```python
from build123d import *

# Parameters (mm, degrees)
SKETCH_1_R      = 1.7
SKETCH_1_R_2    = 2.5
SKETCH_1_R_3    = 2
EXTRUDE_2_DEPTH = 5


with BuildPart() as part:
    # 草图1 → 凸台-拉伸2 (new body)
    with BuildSketch(Plane(origin=(0, 0, 0), x_dir=(1, 0, 0), z_dir=(0, 1, 0))):
        with BuildLine():
            ThreePointArc((-65, 170), (-68.535533906, 168.535533906), (-70, 165))
            Line((-70, 165), (-70, 130))
            Line((-70, 130), (-70, -165))
            ThreePointArc((-70, -165), (-68.535533906, -168.535533906), (-65, -170))
            Line((-65, -170), (65, -170))
            ThreePointArc((65, -170), (68.535533906, -168.535533906), (70, -165))
            Line((70, -165), (70, 165))
            ThreePointArc((70, 165), (68.535533906, 168.535533906), (65, 170))
            Line((65, 170), (0, 170))
            Line((0, 170), (-65, 170))
        make_face()
        with Locations(Location((-62, -158, 0), (0, 0, 270))):
            Circle(SKETCH_1_R, mode=Mode.SUBTRACT)
        with Locations(Location((-48, -158, 0), (0, 0, 270))):
            Circle(SKETCH_1_R, mode=Mode.SUBTRACT)
        with Locations(Location((-62, -142, 0), (0, 0, 270))):
            Circle(SKETCH_1_R, mode=Mode.SUBTRACT)
        with Locations(Location((-48, -142, 0), (0, 0, 270))):
            Circle(SKETCH_1_R, mode=Mode.SUBTRACT)
        with Locations(Location((-35, -160, 0), (0, 0, 270))):
            Circle(SKETCH_1_R_2, mode=Mode.SUBTRACT)
        with Locations(Location((-60, -120, 0), (0, 0, 270))):
            Circle(SKETCH_1_R_3, mode=Mode.SUBTRACT)
        with Locations(Location((-60, -100, 0), (0, 0, 270))):
            Circle(SKETCH_1_R_3, mode=Mode.SUBTRACT)
        with Locations(Location((-40, -100, 0), (0, 0, 270))):
            Circle(SKETCH_1_R_3, mode=Mode.SUBTRACT)
        with Locations(Location((-20, -100, 0), (0, 0, 270))):
            Circle(SKETCH_1_R_3, mode=Mode.SUBTRACT)
        with Locations(Location((-60, -80, 0), (0, 0, 270))):
            Circle(SKETCH_1_R_3, mode=Mode.SUBTRACT)
        with Locations(Location((-60, -60, 0), (0, 0, 270))):
            Circle(SKETCH_1_R_3, mode=Mode.SUBTRACT)
        with Locations(Location((-40, -80, 0), (0, 0, 270))):
            Circle(SKETCH_1_R_3, mode=Mode.SUBTRACT)
        with Locations(Location((-40, -60, 0), (0, 0, 270))):
            Circle(SKETCH_1_R_3, mode=Mode.SUBTRACT)
        with Locations(Location((-60, -40, 0), (0, 0, 270))):
            Circle(SKETCH_1_R_3, mode=Mode.SUBTRACT)
        with Locations(Location((-60, -20, 0), (0, 0, 270))):
            Circle(SKETCH_1_R_3, mode=Mode.SUBTRACT)
        with Locations(Location((-60, 0, 0), (0, 0, 270))):
            Circle(SKETCH_1_R_3, mode=Mode.SUBTRACT)
        with Locations(Location((-40, -40, 0), (0, 0, 270))):
            Circle(SKETCH_1_R_3, mode=Mode.SUBTRACT)
        with Locations(Location((-20, -80, 0), (0, 0, 270))):
            Circle(SKETCH_1_R_3, mode=Mode.SUBTRACT)
        with Locations(Location((-20, -60, 0), (0, 0, 270))):
            Circle(SKETCH_1_R_3, mode=Mode.SUBTRACT)
        with Locations(Location((-20, -40, 0), (0, 0, 270))):
            Circle(SKETCH_1_R_3, mode=Mode.SUBTRACT)
        with BuildLine():
            Line((25, -140), (25, -160))
            ThreePointArc((25, -160), (23.535533906, -163.535533906), (20, -165))
            Line((20, -165), (-20, -165))
            ThreePointArc((-20, -165), (-23.535533906, -163.535533906), (-25, -160))
            Line((-25, -160), (-25, -140))
            ThreePointArc((-25, -140), (-23.535533906, -136.464466094), (-20, -135))
            Line((-20, -135), (20, -135))
            ThreePointArc((20, -135), (23.535533906, -136.464466094), (25, -140))
        make_face(mode=Mode.SUBTRACT)
        with Locations(Location((0, -100, 0), (0, 0, 270))):
            Circle(SKETCH_1_R_3, mode=Mode.SUBTRACT)
        with Locations(Location((20, -100, 0), (0, 0, 270))):
            Circle(SKETCH_1_R_3, mode=Mode.SUBTRACT)
        with Locations(Location((35, -160, 0), (0, 0, 270))):
            Circle(SKETCH_1_R_2, mode=Mode.SUBTRACT)
        with Locations(Location((48, -158, 0), (0, 0, 270))):
            Circle(SKETCH_1_R, mode=Mode.SUBTRACT)
        with Locations(Location((62, -158, 0), (0, 0, 270))):
            Circle(SKETCH_1_R, mode=Mode.SUBTRACT)
        with Locations(Location((48, -142, 0), (0, 0, 270))):
            Circle(SKETCH_1_R, mode=Mode.SUBTRACT)
        with Locations(Location((62, -142, 0), (0, 0, 270))):
            Circle(SKETCH_1_R, mode=Mode.SUBTRACT)
        with Locations(Location((40, -100, 0), (0, 0, 270))):
            Circle(SKETCH_1_R_3, mode=Mode.SUBTRACT)
        with Locations(Location((60, -120, 0), (0, 0, 270))):
            Circle(SKETCH_1_R_3, mode=Mode.SUBTRACT)
        with Locations(Location((60, -100, 0), (0, 0, 270))):
            Circle(SKETCH_1_R_3, mode=Mode.SUBTRACT)
        with Locations(Location((0, -80, 0), (0, 0, 270))):
            Circle(SKETCH_1_R_3, mode=Mode.SUBTRACT)
        with Locations(Location((0, -60, 0), (0, 0, 270))):
            Circle(SKETCH_1_R_3, mode=Mode.SUBTRACT)
        with Locations(Location((20, -80, 0), (0, 0, 270))):
            Circle(SKETCH_1_R_3, mode=Mode.SUBTRACT)
        with Locations(Location((20, -60, 0), (0, 0, 270))):
            Circle(SKETCH_1_R_3, mode=Mode.SUBTRACT)
        with Locations(Location((0, -40, 0), (0, 0, 270))):
            Circle(SKETCH_1_R_3, mode=Mode.SUBTRACT)
        with Locations(Location((20, -40, 0), (0, 0, 270))):
            Circle(SKETCH_1_R_3, mode=Mode.SUBTRACT)
        with Locations(Location((40, -80, 0), (0, 0, 270))):
            Circle(SKETCH_1_R_3, mode=Mode.SUBTRACT)
        with Locations(Location((40, -60, 0), (0, 0, 270))):
            Circle(SKETCH_1_R_3, mode=Mode.SUBTRACT)
        with Locations(Location((60, -80, 0), (0, 0, 270))):
            Circle(SKETCH_1_R_3, mode=Mode.SUBTRACT)
        with Locations(Location((60, -60, 0), (0, 0, 270))):
            Circle(SKETCH_1_R_3, mode=Mode.SUBTRACT)
        with Locations(Location((40, -40, 0), (0, 0, 270))):
            Circle(SKETCH_1_R_3, mode=Mode.SUBTRACT)
        with Locations(Location((60, -40, 0), (0, 0, 270))):
            Circle(SKETCH_1_R_3, mode=Mode.SUBTRACT)
        with Locations(Location((60, -20, 0), (0, 0, 270))):
            Circle(SKETCH_1_R_3, mode=Mode.SUBTRACT)
        with Locations(Location((-60, 20, 0), (0, 0, 270))):
            Circle(SKETCH_1_R_3, mode=Mode.SUBTRACT)
        with Locations(Location((-60, 40, 0), (0, 0, 270))):
            Circle(SKETCH_1_R_3, mode=Mode.SUBTRACT)
        with Locations(Location((-40, 40, 0), (0, 0, 270))):
            Circle(SKETCH_1_R_3, mode=Mode.SUBTRACT)
        with Locations(Location((-60, 60, 0), (0, 0, 270))):
            Circle(SKETCH_1_R_3, mode=Mode.SUBTRACT)
        with Locations(Location((-60, 80, 0), (0, 0, 270))):
            Circle(SKETCH_1_R_3, mode=Mode.SUBTRACT)
        with Locations(Location((-40, 60, 0), (0, 0, 270))):
            Circle(SKETCH_1_R_3, mode=Mode.SUBTRACT)
        with Locations(Location((-40, 80, 0), (0, 0, 270))):
            Circle(SKETCH_1_R_3, mode=Mode.SUBTRACT)
        with Locations(Location((-20, 40, 0), (0, 0, 270))):
            Circle(SKETCH_1_R_3, mode=Mode.SUBTRACT)
        with Locations(Location((-20, 60, 0), (0, 0, 270))):
            Circle(SKETCH_1_R_3, mode=Mode.SUBTRACT)
        with Locations(Location((-20, 80, 0), (0, 0, 270))):
            Circle(SKETCH_1_R_3, mode=Mode.SUBTRACT)
        with Locations(Location((-60, 100, 0), (0, 0, 270))):
            Circle(SKETCH_1_R_3, mode=Mode.SUBTRACT)
        with Locations(Location((-60, 120, 0), (0, 0, 270))):
            Circle(SKETCH_1_R_3, mode=Mode.SUBTRACT)
        with Locations(Location((-40, 100, 0), (0, 0, 270))):
            Circle(SKETCH_1_R_3, mode=Mode.SUBTRACT)
        with Locations(Location((-62, 142, 0), (0, 0, 270))):
            Circle(SKETCH_1_R, mode=Mode.SUBTRACT)
        with Locations(Location((-48, 142, 0), (0, 0, 270))):
            Circle(SKETCH_1_R, mode=Mode.SUBTRACT)
        with Locations(Location((-62, 158, 0), (0, 0, 270))):
            Circle(SKETCH_1_R, mode=Mode.SUBTRACT)
        with Locations(Location((-48, 158, 0), (0, 0, 270))):
            Circle(SKETCH_1_R, mode=Mode.SUBTRACT)
        with Locations(Location((-35, 160, 0), (0, 0, 270))):
            Circle(SKETCH_1_R_2, mode=Mode.SUBTRACT)
        with Locations(Location((-20, 100, 0), (0, 0, 270))):
            Circle(SKETCH_1_R_3, mode=Mode.SUBTRACT)
        with Locations(Location((0, 40, 0), (0, 0, 270))):
            Circle(SKETCH_1_R_3, mode=Mode.SUBTRACT)
        with Locations(Location((20, 40, 0), (0, 0, 270))):
            Circle(SKETCH_1_R_3, mode=Mode.SUBTRACT)
        with Locations(Location((0, 60, 0), (0, 0, 270))):
            Circle(SKETCH_1_R_3, mode=Mode.SUBTRACT)
        with Locations(Location((0, 80, 0), (0, 0, 270))):
            Circle(SKETCH_1_R_3, mode=Mode.SUBTRACT)
        with Locations(Location((20, 60, 0), (0, 0, 270))):
            Circle(SKETCH_1_R_3, mode=Mode.SUBTRACT)
        with Locations(Location((20, 80, 0), (0, 0, 270))):
            Circle(SKETCH_1_R_3, mode=Mode.SUBTRACT)
        with Locations(Location((40, 40, 0), (0, 0, 270))):
            Circle(SKETCH_1_R_3, mode=Mode.SUBTRACT)
        with Locations(Location((60, 0, 0), (0, 0, 270))):
            Circle(SKETCH_1_R_3, mode=Mode.SUBTRACT)
        with Locations(Location((60, 20, 0), (0, 0, 270))):
            Circle(SKETCH_1_R_3, mode=Mode.SUBTRACT)
        with Locations(Location((60, 40, 0), (0, 0, 270))):
            Circle(SKETCH_1_R_3, mode=Mode.SUBTRACT)
        with Locations(Location((40, 60, 0), (0, 0, 270))):
            Circle(SKETCH_1_R_3, mode=Mode.SUBTRACT)
        with Locations(Location((40, 80, 0), (0, 0, 270))):
            Circle(SKETCH_1_R_3, mode=Mode.SUBTRACT)
        with Locations(Location((60, 60, 0), (0, 0, 270))):
            Circle(SKETCH_1_R_3, mode=Mode.SUBTRACT)
        with Locations(Location((60, 80, 0), (0, 0, 270))):
            Circle(SKETCH_1_R_3, mode=Mode.SUBTRACT)
        with Locations(Location((0, 100, 0), (0, 0, 270))):
            Circle(SKETCH_1_R_3, mode=Mode.SUBTRACT)
        with Locations(Location((20, 100, 0), (0, 0, 270))):
            Circle(SKETCH_1_R_3, mode=Mode.SUBTRACT)
        with BuildLine():
            Line((-20, 165), (0, 165))
            Line((0, 165), (20, 165))
            ThreePointArc((20, 165), (23.535533906, 163.535533906), (25, 160))
            Line((25, 160), (25, 140))
            ThreePointArc((25, 140), (23.535533906, 136.464466094), (20, 135))
            Line((20, 135), (-20, 135))
            ThreePointArc((-20, 135), (-23.535533906, 136.464466094), (-25, 140))
            Line((-25, 140), (-25, 160))
            ThreePointArc((-25, 160), (-23.535533906, 163.535533906), (-20, 165))
        make_face(mode=Mode.SUBTRACT)
        with Locations(Location((40, 100, 0), (0, 0, 270))):
            Circle(SKETCH_1_R_3, mode=Mode.SUBTRACT)
        with Locations(Location((60, 100, 0), (0, 0, 270))):
            Circle(SKETCH_1_R_3, mode=Mode.SUBTRACT)
        with Locations(Location((60, 120, 0), (0, 0, 270))):
            Circle(SKETCH_1_R_3, mode=Mode.SUBTRACT)
        with Locations(Location((35, 160, 0), (0, 0, 270))):
            Circle(SKETCH_1_R_2, mode=Mode.SUBTRACT)
        with Locations(Location((48, 142, 0), (0, 0, 270))):
            Circle(SKETCH_1_R, mode=Mode.SUBTRACT)
        with Locations(Location((62, 142, 0), (0, 0, 270))):
            Circle(SKETCH_1_R, mode=Mode.SUBTRACT)
        with Locations(Location((48, 158, 0), (0, 0, 270))):
            Circle(SKETCH_1_R, mode=Mode.SUBTRACT)
        with Locations(Location((62, 158, 0), (0, 0, 270))):
            Circle(SKETCH_1_R, mode=Mode.SUBTRACT)
    extrude(amount=EXTRUDE_2_DEPTH)


solid = part.part
```
Verification items for the finished model (mm, model axes). Coordinates: 2 decimals unless noted, no trailing zeros. Put each result on its own line as item: value.
Item 1: Section check A-A (y = 1.8). Give the number of separate pieces and of enclosed holes in the cut face, then the cut area to 3 significant figures.
Conclusion:
separate pieces: 1
enclosed holes: 88
area: 43,600 mm2
Item 2: Scan lines: line 1 along X through (y, z) = (2.9, 160); line 2 along Z through (x, y) = (14, 2.3); line 3 along X through (y, z) = (2.1, 120). Record each from-to range of solid material in increasing order.
Conclusion:
line 1: x = -70 to -37.5, -32.5 to -25, 25 to 32.5, 37.5 to 70
line 2: z = -170 to -165, -135 to 135, 165 to 170
line 3: x = -70 to -62, -58 to 58, 62 to 70
Item 3: Draft check along Y on faces 1 (the face through (-1, 0, -2)), 2 (the face through (-1, 5, -2)). Enter one of: pulls with the +Y half, pulls with the -Y half, needs draft (parallel to the pull), parting line crosses it, or undercut.
Conclusion:
face 1: pulls with the -Y half
face 2: pulls with the +Y half
